Here's how the part is built. I have some questions about the finished solid (model axes, mm). A direction names the side the tool comes from. Give positions to 0.01 mm unless a question says otherwise; leave off trailing zeros. Write each loop counter-clockwise with the first axis right and the second up, starting at its lowest first coordinate (ties: lowest second). Pieces come first, ordered by that corner, then holes. Notation, with made-up numbers: M 27.25,35.25 L 55.25,35.25 A21 cw 55.25,61.25 Z; hole C 36,-21.75 d7. An arc over 180 degrees is marked long. Answer as CSV lines item,"result". Start each with the question number.
Q1. If I drill on line 1 along Y through (x, z) = (0, 3.8); line 2 along Y through (x, z) = (0, 5.6); line 3 along Y through (x, z) = (0, 6.9), over which ranges is the centre line in solid material (lowest first)?
Q2. Thinking about a two-plate mould opening in X: for faces 4 (the flat face through (-4, -4, 8)), 5 (the flat face through (10.528, -5.965, 2.958)), 6 (the cylindrical face through (-7.7, -13.7, 7.7)), 7 (the flat face through (8.1, 13.8, 3.5)), which applies, +X half, -X half, draft (parallel to the pull), parting line (faces both ways), or undercut?
Q3. Suppose I cut it at B-B (z = 5.5). Write out the boundary of the cut face in (x, y), then the cut area to 3 significant figures.
Q4. Suppose I cut it at A-A (z = 2.5). Write out the boundary of the cut face in (x, y), then the cut area to 3 significant figures.
Q5. Suppose I cut it at C-C (y = 6). Write out the boundary of the cut face in (x, z).
Q6. For pin 1 (2 mm diameter, centred on x = -1.5, z = 6, fed in from -Y); pin 2 (1.8 mm diameter, centred on x = -2.5, z = 2, fed in from -Y); pin 3 (6.5 mm diameter, centred on x = 0, y = 0, fed in from +Z), each with a flat end and sliding along its axis, tell me the tip position at first contact or that it passes through.
Q7. On a 3-axis mill with a long thin cutter (end or side, diameter ignored), from which of +Z, -Z, +X, -X, +Y, -Y can I reach the whole of each face in a straight line? I mean faces 1 (the cylindrical face through (-15.699, -0.129, 7.715)), 2 (the flat face through (10.43, 6.135, 2.958)), 3 (the flat face through (2, -2, 4.8)). Say none if no direction works.
```python
from build123d import *

# Parameters (mm, degrees)
SKIZZE1_R                       = 2.5
AUFSATZ_LINEAR_AUSTRAGEN1_DEPTH = 8
SKIZZE2_R                       = 4.5
SCHNITT_LINEAR_AUSTRAGEN1_DEPTH = 3.2
SKIZZE3_R                       = 8
SCHNITT_LINEAR_AUSTRAGEN2_DEPTH = 6
VERRUNDUNG1_R                   = 1
SKIZZE10_R                      = 8
SCHNITT_LINEAR_AUSTRAGEN3_DEPTH = 2


with BuildPart() as part:
    # Skizze1 → Aufsatz-Linear austragen1 (new body)
    with BuildSketch(Plane.XY):
        Polygon((16, 9.237604307), (0, 18.475208614), (-16, 9.237604307), (-16, -9.237604307), (0, -18.475208614), (16, -9.237604307), align=None)
        Circle(SKIZZE1_R, mode=Mode.SUBTRACT)
    extrude(amount=AUFSATZ_LINEAR_AUSTRAGEN1_DEPTH)

    # Skizze2 → Schnitt-Linear austragen1 (cut)
    with BuildSketch(Plane.XY.offset(8)):
        Circle(SKIZZE2_R)
    extrude(amount=-SCHNITT_LINEAR_AUSTRAGEN1_DEPTH, mode=Mode.SUBTRACT)

    # Skizze3 → Schnitt-Linear austragen2 (cut)
    with BuildSketch(Plane(origin=(0, 0, 0), x_dir=(-1, 0, 0), z_dir=(0, 0, -1))):
        Polygon((13.971876514, 0), (6.985938257, 12.1), (-6.985938257, 12.1), (-13.971876514, 0), (-6.985938257, -12.1), (6.985938257, -12.1), align=None)
        Circle(SKIZZE3_R, mode=Mode.SUBTRACT)
    extrude(amount=-SCHNITT_LINEAR_AUSTRAGEN2_DEPTH, mode=Mode.SUBTRACT)

    # Verrundung1
    verrundung1_edges = [part.edges().sort_by_distance(p)[0] for p in [
        (-8, 13.856406461, 8),
        (-16, 0, 8),
        (-8, -13.856406461, 8),
        (8, -13.856406461, 8),
        (16, 0, 8),
        (8, 13.856406461, 8),
    ]]
    fillet(verrundung1_edges, radius=VERRUNDUNG1_R)

    # Skizze10 → Schnitt-Linear austragen3 (cut)
    with BuildSketch(Plane(origin=(0, 0, 0), x_dir=(-1, 0, 0), z_dir=(0, 0, -1))):
        Circle(SKIZZE10_R)
    extrude(amount=-SCHNITT_LINEAR_AUSTRAGEN3_DEPTH, mode=Mode.SUBTRACT)


solid = part.part
```
Resolved:
1,line 1,"-18.48 to -12.1, -8 to -2.5, 2.5 to 8, 12.1 to 18.48"
1,line 2,"-18.48 to -12.1, -8 to -4.5, 4.5 to 8, 12.1 to 18.48"
1,line 3,"-18.48 to -4.5, 4.5 to 18.48"
2,face 4,"draft"
2,face 5,"undercut"
2,face 6,"-X half"
2,face 7,"+X half"
3,outline,"M -16,-9.24 L 0,-18.48 L 16,-9.24 L 16,9.24 L 0,18.48 L -16,9.24 Z; C 0,0 d16; hole M -13.97,0 L -6.99,-12.1 L 6.99,-12.1 L 13.97,0 L 6.99,12.1 L -6.99,12.1 Z; hole C 0,0 d9"
3,area,"517 mm^2"
4,outline,"M -16,-9.24 L 0,-18.48 L 16,-9.24 L 16,9.24 L 0,18.48 L -16,9.24 Z; C 0,0 d16; hole M -13.97,0 L -6.99,-12.1 L 6.99,-12.1 L 13.97,0 L 6.99,12.1 L -6.99,12.1 Z; hole C 0,0 d5"
4,area,"561 mm^2"
5,outline,"M -16,0 L -10.51,0 L -10.51,6 L -5.29,6 L -5.29,2 L 5.29,2 L 5.29,6 L 10.51,6 L 10.51,0 L 16,0 L 16,7 A1 ccw 15,8 L -15,8 A1 ccw -16,7 Z"
6,pin 1,"y = -18.19"
6,pin 2,"y = -17.55"
6,pin 3,"z = 4.8"
7,face 1,"+Z, -X, +Y, -Y"
7,face 2,"-Z"
7,face 3,"+Z"
